Source: three-view drawing plus pictorial views. Frame: mm from the lowest corner of the part. A direction names the side the tool comes from. Give positions to 0.01 mm unless a question says otherwise; leave off trailing zeros. Loops run counter-clockwise (first coordinate to the right, second up) from the corner with the lowest first, then second, coordinate; pieces in that order, holes last. Notation, with made-up numbers: (38, 20.5) -> (47, 20.5) arc R21 cw to (47, 57.5) -> close; hole circle Ø4 at (66, 42). An arc over 180 degrees is marked (long way). Answer in a Markdown table with one row per item. Add a question column.
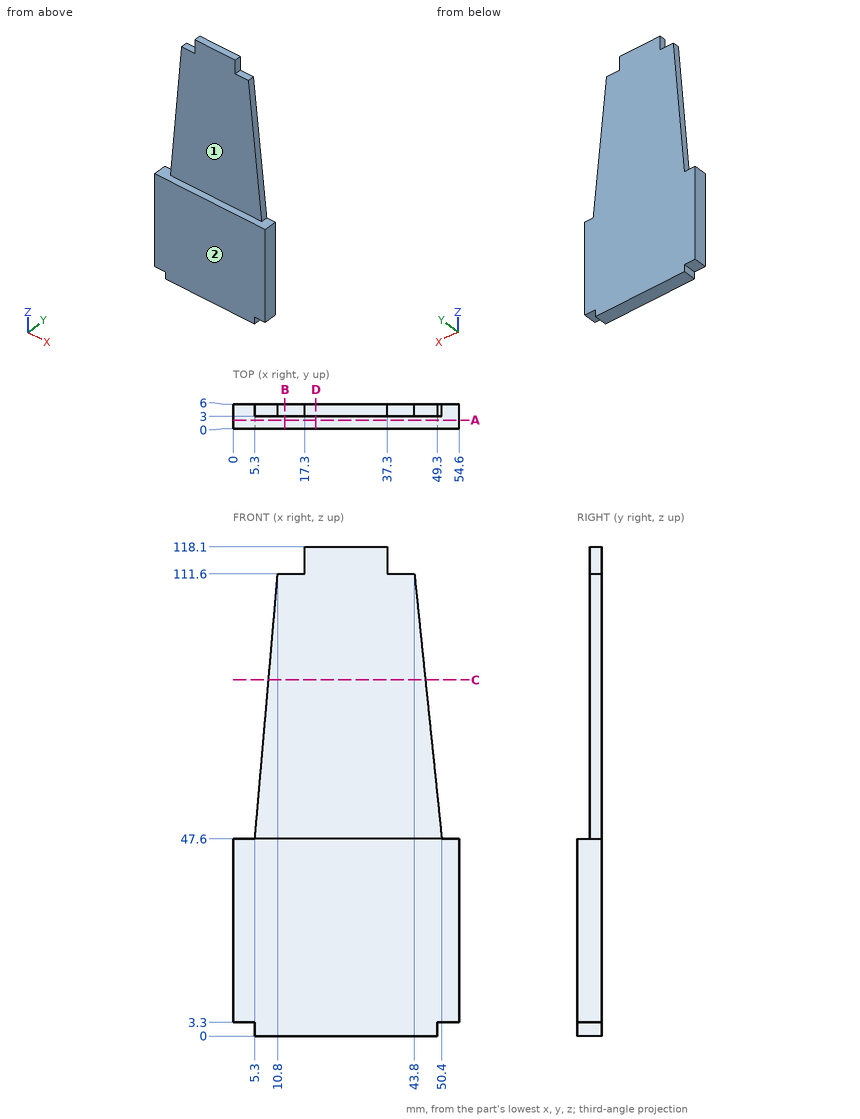
(1) Cut plane B-B on x = 12.5. Return the cut outline in (y, z), then the cut area to 3 significant figures.
(2) Cut plane C-C on z = 86. Return the cut outline in (x, y).
(3) Cut plane A-A on y = 2.1. Return the cut outline in (x, z).
(4) Material intervals for line 1 along Z through (x, y) = (14, 5.45); line 2 along Y through (x, z) = (37, 74); line 3 along Z through (x, y) = (14.5, 2.25), sorted ascending. Write a range as from..to.
(5) Cut plane D-D on x = 20. Return the cut outline in (y, z), then the cut area to 3 significant figures.
(6) Reachability of the marked faces 1 and 2 from +Z, -Z, +X, -X, +Y, -Y: full face, straight path, thin tool, end or side. Return the list, or none.
(7) Pin query (flat end, axial travel): pin 1 Ø2.5 at (x, y) = (3.5, 1.5) entering from -Z; pin 2 Ø1.5 at (x, y) = (13, 4) entering from +Z; pin 3 Ø1 at (y, z) = (2, 1.5) entering from +X. Return the tip coordinate at first contact, or that it passes through.
Answer list:
| question | item | result |
|---|---|---|
| 1 | outline | (0, 0) -> (6, 0) -> (6, 111.6) -> (3, 111.6) -> (3, 47.6) -> (0, 47.6) -> close |
| 1 | area | 478 mm² |
| 2 | outline | (8.6, 3) -> (46.44, 3) -> (46.44, 6) -> (8.6, 6) -> close |
| 3 | outline | (0, 3.3) -> (5.3, 3.3) -> (5.3, 0) -> (49.3, 0) -> (49.3, 3.3) -> (54.6, 3.3) -> (54.6, 47.6) -> (0, 47.6) -> close |
| 4 | line 1 | z = 0..111.6 |
| 4 | line 2 | y = 3..6 |
| 4 | line 3 | z = 0..47.6 |
| 5 | outline | (0, 0) -> (6, 0) -> (6, 118.1) -> (3, 118.1) -> (3, 47.6) -> (0, 47.6) -> close |
| 5 | area | 497 mm² |
| 6 | face 1 | +Z, +X, -X, -Y |
| 6 | face 2 | +Z, -Z, +X, -X, -Y |
| 7 | pin 1 | stops at z = 3.3 |
| 7 | pin 2 | stops at z = 111.6 |
| 7 | pin 3 | stops at x = 49.3 |
